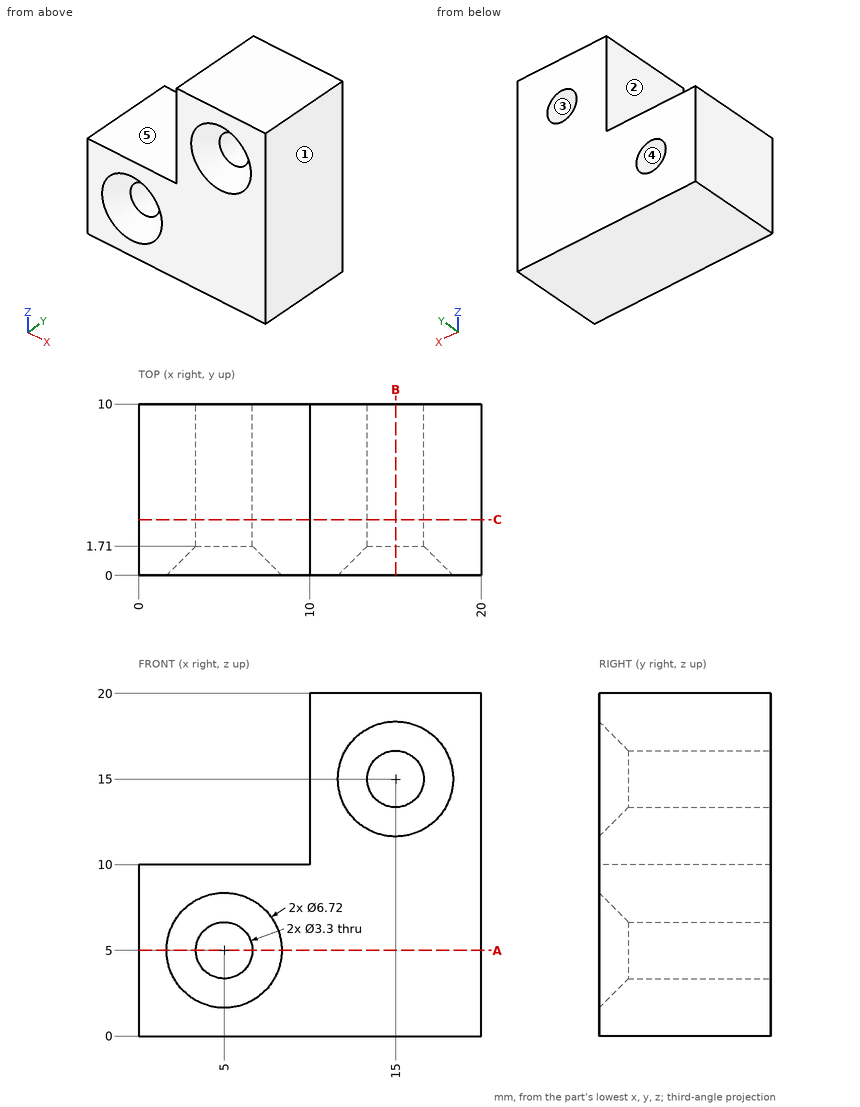
The drawing under review shows one solid part. Ordinate dimensions are in mm from its lowest x, y, z. A direction names the side the tool comes from. Give positions to 0.01 mm unless a question says otherwise; leave off trailing zeros. Loops run counter-clockwise (first coordinate to the right, second up) from the corner with the lowest first, then second, coordinate; pieces in that order, holes last. Notation, with made-up numbers: M -39,47 L -24,47 A17 cw -24,53 Z; hole C -4,-31 d11. An arc over 180 degrees is marked long. Return JSON: item names as keys, results as strings. Group by question number.
Item 1: We need section C-C (y = 3.25). Give the boundary of the cut face in (x, z), and give its area (3 significant figures).
Item 2: Insertion check: pin 1 Ø3 at (x, z) = (5, 5) entering from -Y; pin 2 Ø2 at (y, z) = (5, 12) entering from -X. Each pin has a flat end and moves straight along its axis. Give the tip position at first contact, or say it passes through.
Item 3: Mouldability with a two-part tool opening along X and no side actions: class the marked faces 1, 2 and 3 as released by +X, released by -X, zero draft, split by the parting line, or undercut.
Item 4: We need section A-A (z = 5). Give the boundary of the cut face in (x, y).
Item 5: Tool access review of the marked faces 4 and 5: name each direction out of +Z, -Z, +X, -X, +Y, -Y from which nothing blocks a thin tool from reaching the whole face with its end or side.
Item 6: For probe 1 along X at (y, z) = (8, 5); probe 2 along Z at (x, y) = (5, 7.5); probe 3 along X at (y, z) = (4, 15), list the stretches that pass through material, from the lowest coordinate up.
Item 7: We need section B-B (x = 15). Give the boundary of the cut face in (y, z).
Output:
{
 "1": {"outline": "M 0,0 L 20,0 L 20,20 L 10,20 L 10,10 L 0,10 Z; hole C 5,5 d3.3; hole C 15,15 d3.3", "area": "283 mm^2"},
 "2": {"pin 1": "passes through", "pin 2": "stops at x = 10"},
 "3": {"face 1": "released by +X", "face 2": "released by -X", "face 3": "undercut"},
 "4": {"outline": "M 0,0 L 1.64,0 L 3.35,1.71 L 3.35,10 L 0,10 Z; M 6.65,1.71 L 8.36,0 L 20,0 L 20,10 L 6.65,10 Z"},
 "5": {"face 4": "+Y, -Y", "face 5": "+Z, -X, +Y, -Y"},
 "6": {"probe 1": "x = 0 to 3.35, 6.65 to 20", "probe 2": "z = 0 to 3.35, 6.65 to 10", "probe 3": "x = 10 to 13.35, 16.65 to 20"},
 "7": {"outline": "M 0,0 L 10,0 L 10,13.35 L 1.71,13.35 L 0,11.64 Z; M 0,18.36 L 1.71,16.65 L 10,16.65 L 10,20 L 0,20 Z"}
}
